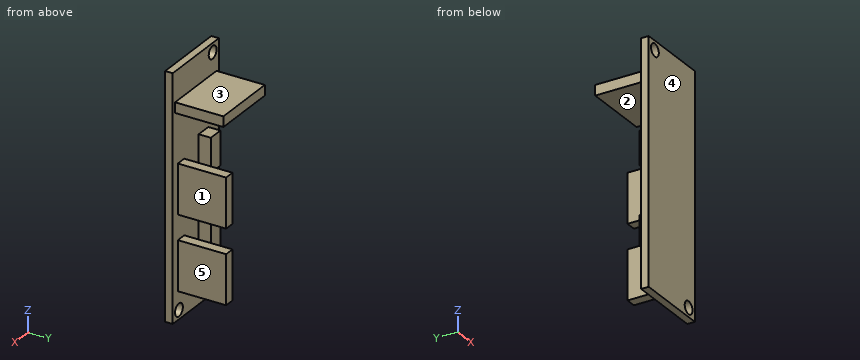
```python
from build123d import *

# Parameters (mm, degrees)
SKETCH1_W           = 19.558
SKETCH1_H           = 63.5
SKETCH1_R           = 1.651
BOSS_EXTRUDE1_DEPTH = 1.984375
SKETCH2_W           = 17.569023062
SKETCH2_H           = 2.702926625
SKETCH2_W_2         = 2.702926625
SKETCH2_H_2         = 12.935434562
BOSS_EXTRUDE3_DEPTH = 12.7
SKETCH2_3_W         = 4.054389937
SKETCH2_3_H         = 7.7226475
SKETCH2_3_H_2       = 8.881044625
BOSS_EXTRUDE4_DEPTH = 3.175


with BuildPart() as part:
    # Sketch1 → Boss-Extrude1 (new body)
    with BuildSketch(Plane(origin=(0, 0, 0), x_dir=(1, 0, 0), z_dir=(0, 1, 0))):
        Rectangle(SKETCH1_W, SKETCH1_H)
        with Locations(Location((7.14375, 29.36875, 0), (0, 0, 270))):
            Circle(SKETCH1_R, mode=Mode.SUBTRACT)
        with Locations(Location((-7.14375, -29.36875, 0), (0, 0, 270))):
            Circle(SKETCH1_R, mode=Mode.SUBTRACT)
    extrude(amount=BOSS_EXTRUDE1_DEPTH)

    # Sketch2 → Boss-Extrude3 (add)
    with BuildSketch(Plane(origin=(0, 1.984375, 0), x_dir=(1, 0, 0), z_dir=(0, 1, 0))):
        with Locations((0, -22.588743937)):
            Rectangle(SKETCH2_W, SKETCH2_H)
        with Locations((6.274651094, 17.955155437)):
            Rectangle(SKETCH2_W_2, SKETCH2_H_2)
        with Locations((6.274651094, -1.447996406)):
            Rectangle(SKETCH2_W_2, SKETCH2_H_2)
    extrude(amount=BOSS_EXTRUDE3_DEPTH)

    # Sketch2_3 → Boss-Extrude4 (add)
    with BuildSketch(Plane(origin=(0, 1.984375, 0), x_dir=(1, 0, 0), z_dir=(0, 1, 0))):
        with Locations((-3.282125188, 13.997298594)):
            Rectangle(SKETCH2_3_W, SKETCH2_3_H)
        with Locations((-3.282125188, -6.853849657)):
            Rectangle(SKETCH2_3_W, SKETCH2_3_H_2)
    extrude(amount=BOSS_EXTRUDE4_DEPTH)


solid = part.part
```
Geometry check sheet. Reference: the model listing, model coordinates, mm. Face numbers are marked on the shaded views. A direction names the side the tool comes from. Give positions to 0.01 mm unless a question says otherwise; leave off trailing zeros. Write each loop counter-clockwise with the first axis right and the second up, starting at its lowest first coordinate (ties: lowest second). Pieces come first, ordered by that corner, then holes.
1) Access from +Z, -Z, +X, -X, +Y, -Y to the whole of each face (thin tool, end or side, straight path). Record for the marked faces 4 and 5.
2) Gauge pin test, flat ends, axial feed: pin 1 (6.5 mm diameter, centred on y = 5.5, z = -17, fed in from +X); pin 2 (3 mm diameter, centred on x = 6.5, y = 9.5, fed in from -Z); pin 3 (2 mm diameter, centred on x = -7.14, z = 29.37, fed in from +Y); pin 4 (1 mm diameter, centred on x = -3, y = 3, fed in from +Z). Record the tip position at first contact, or that the pin passes through.
3) Section check D-D, the plane x = -2.5. Record the boundary of the cut face in (y, z).
4) Section check C-C, the plane x = 6.5. Record the boundary of the cut face in (y, z).
5) Material ranges on L1, parallel to Z at x = 5.25, y = 8.5; L2, parallel to Z at x = -2.5, y = 4.25; L3, parallel to Y at x = -0.75, z = 9, recorded low to high.
6) Section check B-B, the plane z = -13. Record the boundary of the cut face in (x, y).
7) Release check for a two-part mould opening along Z. For the marked faces 1, 2 and 3 record: pulls with the +Z half, pulls with the -Z half, needs draft (parallel to the pull), parting line crosses it, or undercut.
8) Section check A-A, the plane y = 9.75. Record the boundary of the cut face in (x, z), and give its area (3 significant figures).
Computed:
1. face 4: +Z, -Z, +X, -X, -Y
1. face 5: -Z, +X, +Y
2. pin 1: stops at x = 7.63
2. pin 2: stops at z = -24.42
2. pin 3: passes through
2. pin 4: stops at z = 23.94
3. outline: (0, -31.75) - (1.98, -31.75) - (1.98, -17.86) - (5.16, -17.86) - (5.16, -10.14) - (1.98, -10.14) - (1.98, 2.41) - (5.16, 2.41) - (5.16, 11.29) - (1.98, 11.29) - (1.98, 21.24) - (14.68, 21.24) - (14.68, 23.94) - (1.98, 23.94) - (1.98, 31.75) - (0, 31.75) - close
4. outline: (0, -31.75) - (1.98, -31.75) - (1.98, -30.89) - (0, -30.89) - close; (0, -27.85) - (1.98, -27.85) - (1.98, -24.42) - (14.68, -24.42) - (14.68, -11.49) - (1.98, -11.49) - (1.98, -5.02) - (14.68, -5.02) - (14.68, 7.92) - (1.98, 7.92) - (1.98, 21.24) - (14.68, 21.24) - (14.68, 23.94) - (1.98, 23.94) - (1.98, 31.75) - (0, 31.75) - close
5. L1: z = -24.42 to -11.49, -5.02 to 7.92, 21.24 to 23.94
5. L2: z = -17.86 to -10.14, 2.41 to 11.29, 21.24 to 23.94
5. L3: y = 0 to 1.98
6. outline: (-9.78, 0) - (9.78, 0) - (9.78, 1.98) - (7.63, 1.98) - (7.63, 14.68) - (4.92, 14.68) - (4.92, 1.98) - (-1.25, 1.98) - (-1.25, 5.16) - (-5.31, 5.16) - (-5.31, 1.98) - (-9.78, 1.98) - close
7. face 1: needs draft
7. face 2: undercut
7. face 3: pulls with the +Z half
8. outline: (-8.78, 21.24) - (8.78, 21.24) - (8.78, 23.94) - (-8.78, 23.94) - close; (4.92, -24.42) - (7.63, -24.42) - (7.63, -11.49) - (4.92, -11.49) - close; (4.92, -5.02) - (7.63, -5.02) - (7.63, 7.92) - (4.92, 7.92) - close
8. area: 117 mm2
